Input: part model. Units: mm. Frame: model coordinates. Round coordinates to 2 decimals unless told otherwise and drop trailing zeros. Write each loop counter-clockwise with the first axis right and the second up, starting at its lowest first coordinate (ties: lowest second). Pieces come first, ordered by that corner, then holes. Notation, with made-up numbers: (-7.5, -10) -> (19.5, -10) arc R16 ccw to (19.5, 14) -> close; hole circle Ø4 at (89.25, 9). An arc over 180 degrees is marked (long way). Write item = value, one per line. Start each with the question number.
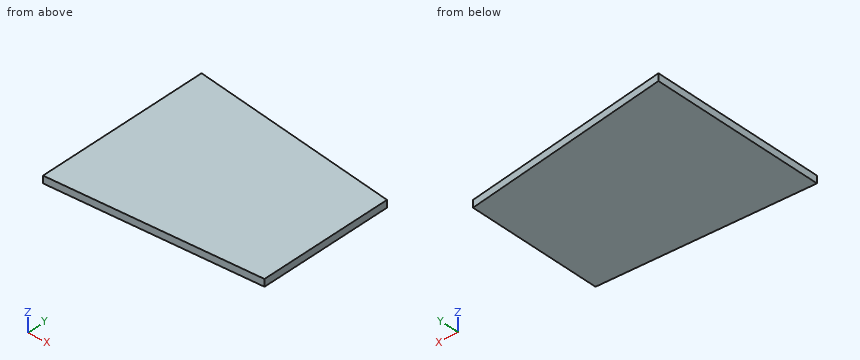
```python
from build123d import *

# Parameters (mm, degrees)
SKETCH006_AS_DRAWN_W                      = 457.2
SKETCH006_AS_DRAWN_H                      = 304.8
EXTRUDE005_DEPTH                          = 7.8
EXTRUDE005_ONTO_SKETCH006_PLACEMENT_ANGLE = 8
EXTRUDE004_DEPTH                          = 152.4


with BuildPart() as hole_depth:
    # Sketch006 as drawn → Extrude005 (new)
    with BuildSketch(Plane.XY):
        Rectangle(SKETCH006_AS_DRAWN_W, SKETCH006_AS_DRAWN_H)
    extrude(amount=-EXTRUDE005_DEPTH)


with BuildPart() as hole_depth_1:
    # Extrude005 onto Sketch006 placement: moved
    add(hole_depth.part.moved(Location((41.07289, 0, 38.415507))).rotate(Axis((41.07289, 0, 38.415507), (0, 1, 0)), EXTRUDE005_ONTO_SKETCH006_PLACEMENT_ANGLE))


with BuildPart() as shallow_hole_volume:
    # Sketch005 → Extrude004 (new body, symmetric)
    with BuildSketch(Plane.XY):
        Polygon((0, 93.031891), (0, -100.091701), (204.503499, -56.19595), (204.503499, 93.031891), align=None)
    extrude(amount=EXTRUDE004_DEPTH, both=True)

    # Common: intersect Hole Depth
    add(hole_depth_1.part, mode=Mode.INTERSECT)


solid = shallow_hole_volume.part
```
1. Section A-A (z = 32). Output: boundary loops of the cut face in (x, y).
2. Section B-B (y = 44). Output: boundary loops of the cut face in (x, z).
3. Pin query (flat end, axial travel): P1, Ø8, axis at x = 166.5, z = 15.5, coming from the -Y side; P2, Ø3, axis at x = 98, z = 22, coming from the -Y side; P3, Ø6, axis at x = 182.5, y = 46.5, coming from the -Z side. Return the tip coordinate at first contact, or that it passes through.
4. Line query: line 1 along Z through (x, y) = (55.5, 46); line 2 along Z through (x, y) = (13.5, 45); line 3 along Y through (x, z) = (82.5, 30). Output: solid intervals per line, ascending.
Check sheet entries:
q1.outline = (30.68, -93.51) -> (86.72, -81.48) -> (86.72, 93.03) -> (30.68, 93.03) -> close
q2.outline = (0, 36.31) -> (204.5, 7.57) -> (204.5, 15.45) -> (0, 44.19) -> close
q3.P1 = -65.21
q3.P2 = -79.34
q3.P3 = 10.24
q4.line_1 = 28.51 to 36.39
q4.line_2 = 34.41 to 42.29
q4.line_3 = -82.38 to 93.03
